Geometry: final body of the model. Coordinates: model frame, mm. Face numbers are marked on the shaded views. A direction names the side the tool comes from. Give positions to 0.01 mm unless a question says otherwise; leave off trailing zeros. Loops run counter-clockwise (first coordinate to the right, second up) from the corner with the lowest first, then second, coordinate; pieces in that order, holes last.
from build123d import *

# Parameters (mm, degrees)
SKETCH1_R           = 0.875
BOSS_EXTRUDE1_DEPTH = 8


with BuildPart() as part:
    # Sketch1 → Boss-Extrude1 (new body)
    with BuildSketch(Plane.XY):
        with BuildLine():
            Line((1.461962708, -0.335656133), (1.194637722, -1.5))
            ThreePointArc((1.194637722, -1.5), (-0.000233431, -3.667871775), (-2.159460582, -4.878294517))
            ThreePointArc((-2.159460582, -4.878294517), (-2.675445647, -4.690989074), (-2.708589557, -4.143060797))
            Line((-2.708589557, -4.143060797), (-1.766378918, -2.5))
            ThreePointArc((-1.766378918, -2.5), (-1.56773594, -2.017435437), (-1.5, -1.5))
            Line((-1.5, -1.5), (-1.5, 0))
            ThreePointArc((-1.5, 0), (0.168902246, 1.490460342), (1.461962708, -0.335656133))
        make_face()
        Circle(SKETCH1_R, mode=Mode.SUBTRACT)
    extrude(amount=BOSS_EXTRUDE1_DEPTH)


solid = part.part
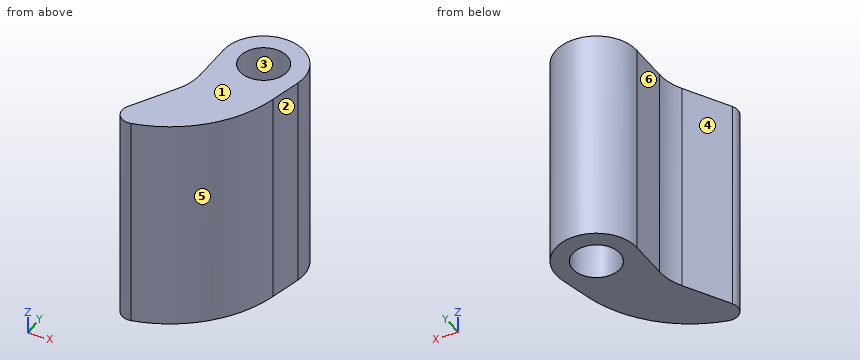
Item 1: Section query C-C on y = 0.5. Return loops of the section in (x, z).
Values follow:
outline: (-1.41, 0) - (-0.72, 0) - (-0.72, 8) - (-1.41, 8) - close; (0.72, 0) - (1.41, 0) - (1.41, 8) - (0.72, 8) - close
Item 2: Draft query along Y for the marked faces 1, 2, 3 and 4. Return one class per face: +Y half, -Y half, draft (parallel to the pull), parting line (faces both ways), or undercut.
Values follow:
face 1: draft
face 2: -Y half
face 3: undercut
face 4: +Y half
Item 3: Ray query, probe 1 along Y at (x, z) = (0, 3.75) (3 decimals); probe 2 along Y at (x, z) = (-0.45, 1); probe 3 along X at (y, z) = (1.25, 3.25). Return the intervals inside material, ascending.
Values follow:
probe 1: y = -3.668 to -0.875, 0.875 to 1.5
probe 2: y = -4.06 to -0.75, 0.75 to 1.43
probe 3: x = -0.83 to 0.83
Item 4: Section query B-B on x = -0.1. Return loops of the section in (y, z).
Values follow:
outline: (-3.77, 0) - (-0.87, 0) - (-0.87, 8) - (-3.77, 8) - close; (0.87, 0) - (1.5, 0) - (1.5, 8) - (0.87, 8) - close
Item 5: Set-up query: the marked faces 5 and 6. Return all of +Z, -Z, +X, -X, +Y, -Y with unobstructed straight access to the full face (end or side cutting, diameter ignored); none if empty.
Values follow:
face 5: +Z, -Z, +X, -Y
face 6: +Z, -Z, -X, +Y
Item 6: Section query D-D on y = -1.25. Return loops of the section in (x, z), plus the area to 3 significant figures.
Values follow:
outline: (-1.5, 0) - (1.25, 0) - (1.25, 8) - (-1.5, 8) - close
area: 22.0 mm2
Item 7: Pin query (flat end, axial travel): pin 1 (2 mm diameter, centred on y = 0.5, z = 5.5, fed in from +X); pin 2 (1.6 mm diameter, centred on y = -0.5, z = 2, fed in from -X). Return the tip coordinate at first contact, or that it passes through.
Values follow:
pin 1: stops at x = 1.5
pin 2: stops at x = -1.5
Item 8: Section query A-A on z = 1.75. Return loops of the section in (x, y) (3 decimals), plus the area to 3 significant figures.
Values follow:
outline: (-2.709, -4.143) arc R0.5 ccw to (-2.159, -4.878) arc R4.509 ccw to (1.195, -1.5) - (1.462, -0.336) arc R1.5 ccw (long way) to (-1.5, 0) - (-1.5, -1.5) arc R2.01 cw to (-1.766, -2.5) - close; hole circle Ø1.75 at (0, 0)
area: 13.2 mm2
